from build123d import *

# Parameters (mm, degrees)
F0_W     = 72
F0_H     = 48
F0_R     = 1.3
F1_DEPTH = 2
F2_SIZE  = 2
F3_R     = 2.05
F4_DEPTH = 25


with BuildPart() as f1:
    # F0 (on Top) → F1 (new body)
    with BuildSketch(Plane.XY):
        Rectangle(F0_W, F0_H)
        with Locations((-23.75, -21)):
            Circle(F0_R, mode=Mode.SUBTRACT)
        with Locations((32.25, -21)):
            Circle(F0_R, mode=Mode.SUBTRACT)
        with Locations((-23.75, 21)):
            Circle(F0_R, mode=Mode.SUBTRACT)
        with Locations((32.25, 21)):
            Circle(F0_R, mode=Mode.SUBTRACT)
    extrude(amount=F1_DEPTH)

    # F2
    f2_edges = [f1.edges().sort_by_distance(p)[0] for p in [
        (-36, -24, 1),
        (36, -24, 1),
        (36, 24, 1),
        (-36, 24, 1),
    ]]
    chamfer(f2_edges, length=F2_SIZE)

    # F3 (on face) → F4 (cut)
    with BuildSketch(Plane.XY.offset(2)):
        with Locations((-30, 0)):
            Circle(F3_R)
        with Locations((30, 0)):
            Circle(F3_R)
    extrude(amount=-F4_DEPTH, mode=Mode.SUBTRACT)


solid = f1.part
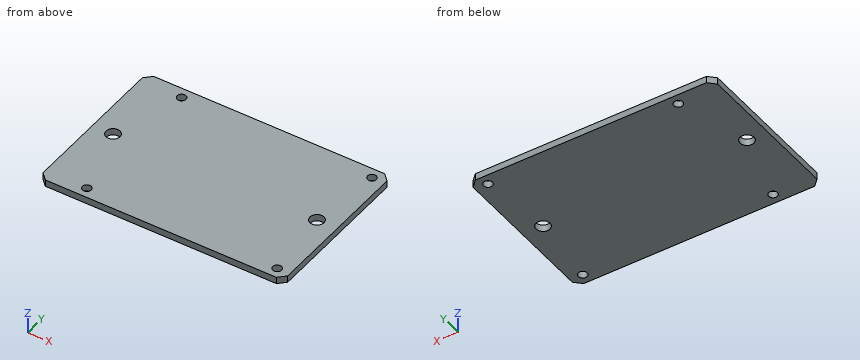
Input: part model. Units: mm. Frame: model coordinates. Coordinates: 2 decimals unless noted, no trailing zeros. Write each loop counter-clockwise with the first axis right and the second up, starting at its lowest first coordinate (ties: lowest second). Pieces come first, ordered by that corner, then holes. Notation, with made-up numbers: M 86.5,-20.5 L 109.5,-20.5 A11 cw 109.5,-6.5 Z; hole C 70,81.25 d10. An arc over 180 degrees is marked long. Answer as a JSON object with one key per item and string values. Group by question number.
(1) Section C-C on z = 0.6. Output: boundary loops of the cut face in (x, y), plus the area to 3 significant figures.
(2) Section A-A on x = 30. Output: boundary loops of the cut face in (y, z).
(3) Section B-B on y = -21. Output: boundary loops of the cut face in (x, z), plus the area to 3 significant figures.
(4) Ray query, line 1 along Y through (x, z) = (-23.75, 1.15); line 2 along Y through (x, z) = (-30, 1.8); line 3 along X through (y, z) = (-1, 0.95). Return the intervals inside material, ascending. Write a range as [from, to].
Result set:
{
 "1": {"outline": "M -36,-22 L -34,-24 L 34,-24 L 36,-22 L 36,22 L 34,24 L -34,24 L -36,22 Z; hole C -30,0 d4.1; hole C -23.75,-21 d2.6; hole C -23.75,21 d2.6; hole C 30,0 d4.1; hole C 32.25,-21 d2.6; hole C 32.25,21 d2.6", "area": "3,400 mm2"},
 "2": {"outline": "M -24,0 L -2.05,0 L -2.05,2 L -24,2 Z; M 2.05,0 L 24,0 L 24,2 L 2.05,2 Z"},
 "3": {"outline": "M -36,0 L -25.05,0 L -25.05,2 L -36,2 Z; M -22.45,0 L 30.95,0 L 30.95,2 L -22.45,2 Z; M 33.55,0 L 36,0 L 36,2 L 33.55,2 Z", "area": "134 mm2"},
 "4": {"line 1": "y = [-24, -22.3], [-19.7, 19.7], [22.3, 24]", "line 2": "y = [-24, -2.05], [2.05, 24]", "line 3": "x = [-36, -31.79], [-28.21, 28.21], [31.79, 36]"}
}
